Read the model definition and answer for the solid it produces. Units are mm, in the model's axes. A direction names the side the tool comes from. Coordinates: 2 decimals unless noted, no trailing zeros. Write each loop counter-clockwise with the first axis right and the second up, starting at its lowest first coordinate (ties: lowest second). Pieces come first, ordered by that corner, then holes.
1) The part is cut by section A-A (z = -3.5). Determine the outline of the cut face in (x, y), then the cut area to 3 significant figures.
2) Find the intervals of material crossed by line 1 (Y direction, x = -111.9, z = 0.65); line 2 (Y direction, x = 100.65, z = 0.6); line 3 (X direction, y = 148.3, z = 1), in increasing order.
3) Which of the six approach directions +Z, -Z, +X, -X, +Y, -Y give full straight-line access (tool end or side, diameter ignored) to faces 1 (the face through (-109.5, 72, -4)), 2 (the face through (-113, 146.4, -4)), 3 (the face through (-113, 0, -3))?
4) The part is cut by section C-C (x = -66.5). Determine the outline of the cut face in (y, z).
5) Determine the mould class of faces 4 (the face through (104, 142.5, -4)), 5 (the face through (-113, 160.5, -4)), 6 (the face through (98.25, 171, -4)) for opening direction Y: +Y half, -Y half, draft (parallel to the pull), parting line (faces both ways), or undercut.
6) The part is cut by section B-B (y = 22). Determine the outline of the cut face in (x, z), then the cut area to 4 significant figures.
7) Each of these flat-tipped pins is pushed along its axis until it touches: pin 1 Ø1.5 at (x, z) = (43, -5.5) entering from -Y; pin 2 Ø3 at (x, y) = (100.65, 156.7) entering from -Z; pin 3 Ø0.8 at (x, z) = (15, 0.5) entering from -Y. Where does it stop, or does it pass through?
Autodesk Inventor part; units mm, degrees
ref_plane "YZ Plane" through (0, 0, 0) normal (1, 0, 0) x (0, 1, 0)
ref_plane "XZ Plane" through (0, 0, 0) normal (0, 1, 0) x (-1, 0, 0)
ref_plane "XY Plane" through (0, 0, 0) normal (0, 0, 1) x (1, 0, 0)
sketch "Boceto1" plane through (0, 0, 0) normal (0, 0, 1) x (1, 0, 0)
  circle A0 centre (100.65, -156.7) radius 1.65
  circle A1 centre (100.65, -148.3) radius 1.65
  circle A2 centre (100.65, 156.7) radius 1.65
  circle A3 centre (100.65, 148.3) radius 1.65
  line L0 (97.75, 145) -> (105.25, 145)
  line L1 (105.25, 145) -> (105.25, 160)
  line L2 (105.25, 160) -> (97.75, 160)
  line L3 (97.75, 160) -> (97.75, 180)
  line L4 (97.75, 180) -> (-109, 180)
  line L5 (-109, 160) -> (-115.3, 160)
  line L6 (-109, -160) -> (-109, -180)
  line L7 (-115.3, 146.9) -> (-109, 146.9)
  line L8 (-109, -146.9) -> (-115.3, -146.9)
  line L9 (-109, 180) -> (-109, 160)
  line L10 (-115.3, -160) -> (-109, -160)
  line L11 (-109, -180) -> (97.75, -180)
  line L12 (97.75, -180) -> (97.75, -160)
  line L13 (97.75, -160) -> (105.25, -160)
  line L14 (105.25, -160) -> (105.25, -145)
  line L15 (105.25, -145) -> (97.75, -145)
  line L16 (97.75, -145) -> (97.75, -142)
  line L17 (97.75, -142) -> (109, -142)
  line L18 (109, -142) -> (109, 142)
  line L19 (109, 142) -> (97.75, 142)
  line L20 (97.75, 142) -> (97.75, 145)
  line L21 (109, 180) -> (97.75, 180)
  line L22 (-109, -160) -> (-109, -180)
  line L23 (-109, -180) -> (-102.7, -180)
  line L24 (-109, -180) -> (109, -180)
  line L25 (109, -180) -> (109, 180)
  line L26 (109, 180) -> (-109, 180)
  line L27 (111, 142) -> (111, 180)
  line L28 (109, 182) -> (97.75, 182)
  line L29 (-109, -182) -> (-102.7, -182)
  line L30 (-111, -182) -> (111, -182)
  line L31 (111, -182) -> (111, 182)
  line L32 (111, 182) -> (-111, 182)
  circle A4 centre (-111.9, -156.3) radius 1.2
  circle A5 centre (-111.9, -150.6) radius 1.2
  circle A6 centre (-111.9, 156.3) radius 1.2
  circle A7 centre (-111.9, 150.6) radius 1.2
  line L33 (-115.3, 160) -> (-115.3, 146.9)
  line L34 (-109, 146.9) -> (-109, -146.9)
  line L35 (-115.3, -146.9) -> (-115.3, -160)
  line L36 (-109, 180) -> (-115.3, 180)
  line L37 (-109, -180) -> (-115.3, -180)
  line L38 (-115.3, 180) -> (109, 180)
  line L39 (109, 180) -> (109, -180)
  line L40 (109, -180) -> (-115.3, -180)
  line L41 (-115.3, -180) -> (-115.3, 180)
  line L42 (-117.3, 180) -> (-117.3, -182)
  line L43 (-117.3, -182) -> (109, -182)
  line L44 (-115.3, 182) -> (111, 182)
  line L45 (111, 182) -> (111, -180)
  line L46 (-117.3, 180) -> (-117.3, 182)
  line L47 (-117.3, 182) -> (-115.3, 182)
  point P0 (0, 0)
  dimension "d1" = 2
  dimension "d3" = 2
  dimension "d20" = 2
  dimension "d21" = 2
extrude "Extrusión1" add sketch "Boceto1" against normal blind 7.5 contours L0 L1 L2 L3 L21 L25 L19 L20 | L25 L24 L12 L13 L14 L15 L16 L17 | L9 L5 L41 L36 | L37 L41 L10 L6 | L7 L34 L8 L41 | L31 L30 L29 L43 L42 L46 L47 L44 L32 L28 L27
sketch "Boceto2" plane through (0, 0, 0) normal (0, 0, 1) x (1, 0, 0)
  line L0 (-117.3, -182) -> (111, -182)
  line L1 (111, -182) -> (111, 182)
  line L2 (111, 182) -> (-117.3, 182)
  line L3 (90.8, 170.8) -> (90.8, -176)
  line L4 (90.8, 170.8) -> (90.8, -176)
  line L5 (-19.4789, -176) -> (90.8, -176)
  line L6 (90.8, -176) -> (-99.7, -176)
  line L7 (-99.7, -176) -> (-99.7, 170.8)
  line L8 (-99.7, 170.8) -> (90.8, 170.8)
  line L9 (-117.3, 182) -> (-117.3, -182)
  line L10 (-105.5008, -176) -> (-99.7, -176)
  line L11 (-99.7, 170.8) -> (-105.5008, 170.8)
  line L12 (-109, 160) -> (-109, 180)
  line L13 (-109, 170.8) -> (-105, 170.8)
  line L14 (-105, 170.8) -> (-105, -176)
  point P0 (0, 0)
  dimension "d33" = 4
extrude "Extrusión2" add sketch "Boceto2" along normal blind 1.5
sketch "Boceto3" plane through (-111, -182, -7.5) normal (0, -1, 0) x (1, 0, 0)
  line L0 (222, 0) -> (-6.3, 0)
  line L1 (222, 0) -> (222, 9)
  line L2 (-6.3, 9) -> (222, 9)
  line L3 (-6.3, 0) -> (-6.3, 9)
  point P0 (111, 7.5)
extrude "Extrusión3" add sketch "Boceto3" along normal blind 5.2
sketch "Boceto5" plane through (0, 0, 1.5) normal (0, 0, 1) x (1, 0, 0)
  circle A0 centre (100.65, -156.7) radius 1.65
  circle A1 centre (100.65, -148.3) radius 1.65
  circle A2 centre (100.65, 156.7) radius 1.65
  circle A3 centre (100.65, 148.3) radius 1.65
  line L0 (97.75, 145) -> (105.25, 145)
  line L1 (105.25, 145) -> (105.25, 160)
  line L2 (105.25, 160) -> (97.75, 160)
  line L3 (97.75, 160) -> (97.75, 180)
  line L4 (97.75, 180) -> (-109, 180)
  line L5 (-109, 160) -> (-115.3, 160)
  line L6 (-109, -160) -> (-109, -180)
  line L7 (-115.3, 146.9) -> (-109, 146.9)
  line L8 (-109, -146.9) -> (-115.3, -146.9)
  line L9 (-109, 180) -> (-109, 160)
  line L10 (-115.3, -160) -> (-109, -160)
  line L11 (-109, -180) -> (97.75, -180)
  line L12 (97.75, -180) -> (97.75, -160)
  line L13 (97.75, -160) -> (105.25, -160)
  line L14 (105.25, -160) -> (105.25, -145)
  line L15 (105.25, -145) -> (97.75, -145)
  line L16 (97.75, -145) -> (97.75, -142)
  line L17 (97.75, -142) -> (109, -142)
  line L18 (109, -142) -> (109, 142)
  line L19 (109, 142) -> (97.75, 142)
  line L20 (97.75, 142) -> (97.75, 145)
  circle A4 centre (-111.9, -156.3) radius 1.2
  circle A5 centre (-111.9, -150.6) radius 1.2
  circle A6 centre (-111.9, 156.3) radius 1.2
  circle A7 centre (-111.9, 150.6) radius 1.2
  line L21 (-115.3, 160) -> (-115.3, 146.9)
  line L22 (-109, 146.9) -> (-109, -146.9)
  line L23 (-115.3, -146.9) -> (-115.3, -160)
  point P0 (0, 0)
hole "Agujero1" at (100.65, 148.3, 1.5) at (100.65, 156.7, 1.5) at (100.65, -156.7, 1.5) at (100.65, -148.3, 1.5) at (-111.9, -156.3, 1.5) at (-111.9, -150.6, 1.5) at (-111.9, 150.6, 1.5) at (-111.9, 156.3, 1.5) direction (0, 0, -1) diameter 2.4 end through all
sketch "Boceto6" plane through (0, 0, -7.5) normal (0, 0, -1) x (-1, 0, 0)
  line L0 (117.3, 182) -> (-111, 182)
  line L1 (-111, 182) -> (-111, -187.2)
  line L2 (117.3, -187.2) -> (-111, -187.2)
  line L3 (117.3, 182) -> (117.3, -187.2)
  line L4 (-97.75, 160) -> (-97.75, 180)
  line L5 (-97.75, 180) -> (109, 180)
  line L6 (109, 180) -> (109, 160)
  line L7 (109, 160) -> (115.3, 160)
  line L8 (115.3, 160) -> (115.3, 146.9)
  line L9 (115.3, 146.9) -> (109, 146.9)
  line L10 (109, 146.9) -> (109, -146.9)
  line L11 (109, -146.9) -> (115.3, -146.9)
  line L12 (115.3, -146.9) -> (115.3, -160)
  line L13 (115.3, -160) -> (109, -160)
  line L14 (109, -160) -> (109, -180)
  line L15 (109, -180) -> (-97.75, -180)
  line L16 (-97.75, -180) -> (-97.75, -160)
  line L17 (-97.75, -160) -> (-105.25, -160)
  line L18 (-105.25, -160) -> (-105.25, -145)
  line L19 (-105.25, -145) -> (-97.75, -145)
  line L20 (-97.75, -145) -> (-97.75, -142)
  line L21 (-97.75, -142) -> (-109, -142)
  line L22 (-109, -142) -> (-109, 142)
  line L23 (-109, 142) -> (-97.75, 142)
  line L24 (-97.75, 142) -> (-97.75, 145)
  line L25 (-97.75, 145) -> (-105.25, 145)
  line L26 (-105.25, 145) -> (-105.25, 160)
  line L27 (-105.25, 160) -> (-97.75, 160)
  line L28 (117.3, 182) -> (117.3, -187.2)
  line L29 (117.3, 182) -> (-111, 182)
  line L30 (-111, 182) -> (-111, -187.2)
  line L31 (117.3, -187.2) -> (-111, -187.2)
  line L32 (109.5, 160.5) -> (109.5, 180.5)
  line L33 (109.5, 180.5) -> (-98.25, 180.5)
  line L34 (-98.25, 180.5) -> (-98.25, 160.5)
  line L35 (-98.25, 160.5) -> (-105.75, 160.5)
  line L36 (-105.75, 160.5) -> (-105.75, 144.5)
  line L37 (-105.75, 144.5) -> (-98.25, 144.5)
  line L38 (-98.25, 144.5) -> (-98.25, 142.5)
  line L39 (-98.25, 142.5) -> (-109.5, 142.5)
  line L40 (-109.5, 142.5) -> (-109.5, -142.5)
  line L41 (-109.5, -142.5) -> (-98.25, -142.5)
  line L42 (-98.25, -142.5) -> (-98.25, -144.5)
  line L43 (-98.25, -144.5) -> (-105.75, -144.5)
  line L44 (-105.75, -144.5) -> (-105.75, -160.5)
  line L45 (-105.75, -160.5) -> (-98.25, -160.5)
  line L46 (-98.25, -160.5) -> (-98.25, -180.5)
  line L47 (-98.25, -180.5) -> (109.5, -180.5)
  line L48 (109.5, -180.5) -> (109.5, -160.5)
  line L49 (109.5, -160.5) -> (115.8, -160.5)
  line L50 (115.8, -160.5) -> (115.8, -146.4)
  line L51 (115.8, -146.4) -> (109.5, -146.4)
  line L52 (109.5, -146.4) -> (109.5, 146.4)
  line L53 (109.5, 146.4) -> (115.8, 146.4)
  line L54 (115.8, 146.4) -> (115.8, 160.5)
  line L55 (115.8, 160.5) -> (109.5, 160.5)
  dimension "d22" = 0.5
extrude "Extrusión4" cut sketch "Boceto6" against normal blind 7.5 contours L55 L54 L53 L52 L51 L50 L49 L48 L47 L46 L45 L44 L43 L42 L41 L40 L39 L38 L37 L36 L35 L34 L33 L32
fillet "Empalme1" radius 2 5 edges at (-117.3, 182, 0.75) (-117.3, 182, -3.75) (111, 182, -3) (111, -187.2, -3) (-117.3, -187.2, -3)
sketch "Boceto7" plane through (0, 0, -7.5) normal (0, 0, -1) x (-1, 0, 0)
  arc A0 (117.3, 7) -> (114.3, 10) centre (114.3, 7) ccw
  line L0 (114.3, 10) -> (100.3, 10)
  arc A1 (100.3, 10) -> (97.3, 7) centre (100.3, 7) ccw
  line L1 (97.3, 7) -> (97.3, -7)
  arc A2 (97.3, -7) -> (100.3, -10) centre (100.3, -7) ccw
  line L2 (100.3, -10) -> (114.3, -10)
  arc A3 (114.3, -10) -> (117.3, -7) centre (114.3, -7) ccw
  line L3 (117.3, -7) -> (117.3, 7)
  circle A4 centre (103.3, -5) radius 1
  circle A5 centre (113.3, 5) radius 1
  circle A6 centre (103.3, 5) radius 1
  circle A7 centre (113.3, -5) radius 1
  circle A8 centre (113.3, 5) radius 1
  point P0 (0, 0)
hole "Agujero2" at (-113.3, 5, -7.5) at (-113.3, -5, -7.5) direction (0, 0, 1) diameter 3 depth 6
split "Dividir4" plane through (0, 0, 0) removes the side toward (0, -1, 0)
Reported:
1. outline: (-117.3, 0) - (-109.5, 0) - (-109.5, 146.4) - (-115.8, 146.4) - (-115.8, 160.5) - (-109.5, 160.5) - (-109.5, 180.5) - (98.25, 180.5) - (98.25, 160.5) - (105.75, 160.5) - (105.75, 144.5) - (98.25, 144.5) - (98.25, 142.5) - (109.5, 142.5) - (109.5, 0) - (111, 0) - (111, 180) arc R2 ccw to (109, 182) - (-115.3, 182) arc R2 ccw to (-117.3, 180) - close; hole circle Ø3 at (-113.3, 5)
1. area: 2,230 mm2
2. line 1: y = 0 to 149.4, 151.8 to 155.1, 157.5 to 182
2. line 2: y = 0 to 147.1, 149.5 to 155.5, 157.9 to 182
2. line 3: x = -117.3 to -105, 90.8 to 99.45, 101.85 to 111
3. face 1: -Z, -Y
3. face 2: -Z
3. face 3: +Z, -Z, +X, -X, -Y
4. outline: (170.8, 0) - (180.5, 0) - (180.5, -7.5) - (182, -7.5) - (182, 1.5) - (170.8, 1.5) - close
5. face 4: -Y half
5. face 5: undercut
5. face 6: draft
6. outline: (-117.3, -7.5) - (-109.5, -7.5) - (-109.5, 0) - (-105, 0) - (-105, 1.5) - (-117.3, 1.5) - close; (90.8, 0) - (109.5, 0) - (109.5, -7.5) - (111, -7.5) - (111, 1.5) - (90.8, 1.5) - close
6. area: 118.5 mm2
7. pin 1: stops at y = 180.5
7. pin 2: stops at z = 0
7. pin 3: stops at y = 170.8
